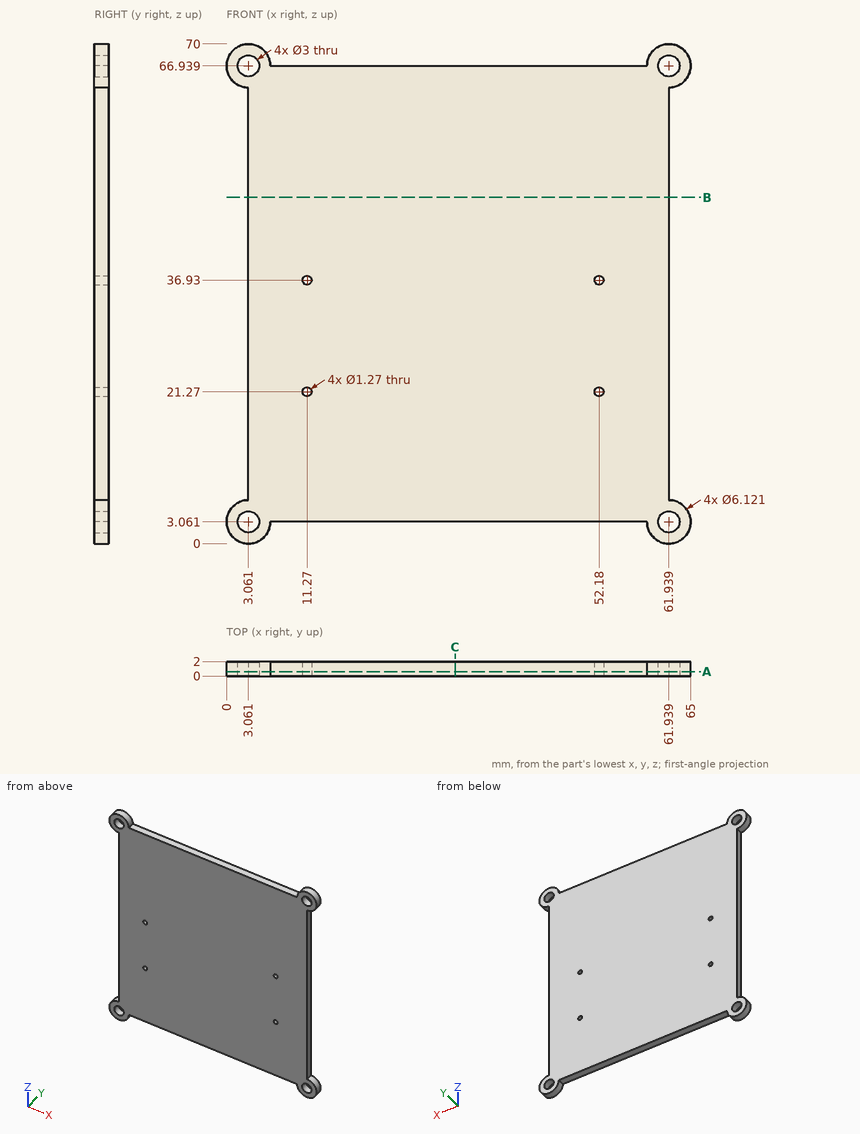
The figure shows three views and two pictorial views of one solid part (mm, origin at its lowest corner). Answer the questions. Round coordinates to 2 decimals unless told otherwise and drop trailing zeros. Order: outer loops, then holes, each group sorted by start corner. A loop starts at its lowest first (then second) coordinate and runs counter-clockwise, first axis right, second up.
Q1. Given pin 1 Ø1 at (x, y) = (23.5, 1.5) entering from -Z; pin 2 Ø1 at (y, z) = (1.5, 43.5) entering from -X; pin 3 Ø1 at (y, z) = (0.5, 37.5) entering from +X, each flat-ended and moving along its own axis, determine where each tip first touches the part or whether it passes through.
Solution:
pin 1: stops at z = 3.06
pin 2: stops at x = 3.06
pin 3: stops at x = 61.94
Q2. A cutting plane is placed at C-C, the plane x = 32. Determine the outline of the cut face in (y, z).
Solution:
outline: (0, 3.06) - (2, 3.06) - (2, 66.94) - (0, 66.94) - close
Q3. A cutting plane is placed at B-B, the plane z = 48.5. Determine the outline of the cut face in (x, y), then the cut area to 3 significant figures.
Solution:
outline: (3.06, 0) - (61.94, 0) - (61.94, 2) - (3.06, 2) - close
area: 118 mm2
Q4. A cutting plane is placed at A-A, the plane y = 0.6. Count the separate pieces of the cut face and the enclosed holes in it, then the cut area to 3 significant figures.
Solution:
separate pieces: 1
enclosed holes: 8
area: 3,820 mm2
Q5. Find the intervals of material crossed by line 1 along Z through (x, y) = (52.18, 1) (1 decimal); line 2 along X through (y, z) = (1.5, 36.93) (1 decimal); line 3 along X through (y, z) = (0.9, 66), in increasing order.
Solution:
line 1: z = 3.1 to 20.6, 21.9 to 36.3, 37.6 to 66.9
line 2: x = 3.1 to 10.6, 11.9 to 51.5, 52.8 to 61.9
line 3: x = 0.15 to 1.89, 4.23 to 60.77, 63.11 to 64.85
